Check sheet for the modelled part. Datum: model origin and axes. Units: mm. A direction names the side the tool comes from. Give positions to 0.01 mm unless a question says otherwise; leave off trailing zeros. Order: outer loops, then holes, each group sorted by start corner. A loop starts at its lowest first (then second) coordinate and runs counter-clockwise, first axis right, second up. Notation, with made-up numbers: (33.5, -31) -> (37.5, -31) arc R23 cw to (37.5, -19) -> close; hole circle Ø2 at (19, 12.5). An arc over 180 degrees is marked (long way). Answer in a Markdown table with one row per item. Add a question column.
(1) Cross-section at B-B (y = 0). Record the cut outline in (x, z).
(2) Release check for a two-part mould opening along Z. For faces 6 (the face through (-4.3, 4.5, 4.5)), 7 (the face through (0, 8, 3)), 8 (the face through (0.56, 6.14, 7)) record: released by +Z, released by -Z, zero draft, split by the parting line, or undercut.
(3) Cross-section at A-A (z = 3.5). Record the cut outline in (x, y).
(4) Set-up check for faces 1 (the face through (0, 4.5, -7)), 2 (the face through (-1.25, 7, 3)), 3 (the face through (7, 1.25, 3)), 4 (the face through (0, -1.25, 2)), 5 (the face through (-4.9, 5, 5.8)): record each of +Z, -Z, +X, -X, +Y, -Y from which the full face is reachable in a straight line by a thin tool's end or side.
(5) Cross-section at D-D (x = 0). Record the cut outline in (y, z), then the cut area to 3 significant figures.
(6) Cross-section at C-C (x = -6.5). Record the cut outline in (y, z), then the cut area to 3 significant figures.
(7) Go/stop test with flat-tipped pins: pin 1 (3 mm diameter, centred on x = -5.5, y = 5, fed in from -Z); pin 2 (2.5 mm diameter, centred on x = -0.5, y = 7.5, fed in from -Z); pin 3 (1.8 mm diameter, centred on x = 0.5, z = -8.5, fed in from +Y). Record where each tip stops, or that it passes through.
(8) Thickness scan on L1, parallel to Z at x = 4, y = 3.75; L2, parallel to Z at x = 3, y = 5.75; L3, parallel to Z at x = 2.5, y = 3.25. Record the ranges inside material, lowest first. Write a range as [from, to].
```python
from build123d import *
from build123d.topology import SkipClean

# Parameters (mm, degrees)
BOSS_EXTRUDE1_DEPTH = 7
BOSS_EXTRUDE2_DEPTH = 16
BOSS_EXTRUDE3_START = -16
BOSS_EXTRUDE3_DEPTH = 2.5
BOSS_EXTRUDE4_START = -5
BOSS_EXTRUDE4_DEPTH = 2.5
CUT_EXTRUDE1_START  = -7
SKETCH7_R           = 7.581765893
CUT_EXTRUDE1_DEPTH  = 7
BOSS_EXTRUDE5_START = 3
BOSS_EXTRUDE5_DEPTH = 3
BOSS_EXTRUDE6_DEPTH = 8
BOSS_EXTRUDE7_DEPTH = 8


with BuildPart() as part:
    # Sketch1 → Boss-Extrude1 (new body)
    with BuildSketch(Plane.XY):
        with BuildLine():
            Line((8, 1.25), (5.868347297, 1.25))
            ThreePointArc((5.868347297, 1.25), (4.242640687, 4.242640687), (1.25, 5.868347297))
            Line((1.25, 5.868347297), (1.25, 8))
            Line((1.25, 8), (-1.25, 8))
            Line((-1.25, 8), (-1.25, 5.868347297))
            ThreePointArc((-1.25, 5.868347297), (-4.242640687, 4.242640687), (-5.868347297, 1.25))
            Line((-5.868347297, 1.25), (-8, 1.25))
            Line((-8, 1.25), (-8, -1.25))
            Line((-8, -1.25), (8, -1.25))
            Line((8, -1.25), (8, 1.25))
        make_face()
    extrude(amount=BOSS_EXTRUDE1_DEPTH)

    # Sketch3 → Boss-Extrude2 (add)
    with BuildSketch(Plane.XY.offset(7)):
        with BuildLine():
            Line((-5.868347297, -1.25), (5.868347297, -1.25))
            ThreePointArc((5.868347297, -1.25), (0, 6), (-5.868347297, -1.25))
        make_face()
    extrude(amount=BOSS_EXTRUDE2_DEPTH)

    # Sketch5 → Boss-Extrude3 (add)
    with BuildSketch(Plane.XY.offset(23).offset(BOSS_EXTRUDE3_START)):
        with BuildLine():
            Line((-6.887488657, -1.25), (6.887488657, -1.25))
            ThreePointArc((6.887488657, -1.25), (0, 7), (-6.887488657, -1.25))
        make_face()
    extrude(amount=-BOSS_EXTRUDE3_DEPTH)

    # Sketch6 → Boss-Extrude4 (add)
    with BuildSketch(Plane.XY.offset(23).offset(BOSS_EXTRUDE4_START)):
        with BuildLine():
            Line((-6.887488657, -1.25), (6.887488657, -1.25))
            ThreePointArc((6.887488657, -1.25), (0, 7), (-6.887488657, -1.25))
        make_face()
    extrude(amount=-BOSS_EXTRUDE4_DEPTH)

    # Sketch7 → Cut-Extrude1 (cut)
    with BuildSketch(Plane.XY.offset(23).offset(CUT_EXTRUDE1_START)):
        Circle(SKETCH7_R)
        with BuildLine():
            Line((-4.841229183, -1.25), (4.841229183, -1.25))
            ThreePointArc((4.841229183, -1.25), (0, 5), (-4.841229183, -1.25))
        make_face(mode=Mode.SUBTRACT)
    extrude(amount=-CUT_EXTRUDE1_DEPTH, mode=Mode.SUBTRACT)

    # Sketch8 → Boss-Extrude5 (add)
    with SkipClean():  # the faces are left unmerged after this step: merging them gives an invalid solid
        with BuildSketch(Plane(origin=(0, 0, 0), x_dir=(-1, 0, 0), z_dir=(0, 0, -1)).offset(BOSS_EXTRUDE5_START)):
            with BuildLine():
                Line((-5.868347297, -1.25), (5.868347297, -1.25))
                ThreePointArc((5.868347297, -1.25), (0, 6), (-5.868347297, -1.25))
            make_face()
        extrude(amount=-BOSS_EXTRUDE5_DEPTH)

    # Sketch9 → Boss-Extrude6 (add)
    with SkipClean():  # the faces are left unmerged after this step: merging them gives an invalid solid
        with BuildSketch(Plane(origin=(0, 0, -3), x_dir=(-1, 0, 0), z_dir=(0, 0, -1))):
            with BuildLine():
                Line((-3.588523373, -1.25), (3.588523373, -1.25))
                ThreePointArc((3.588523373, -1.25), (3.321506513, 1.845967087), (0.833333333, 3.707499906))
                Line((0.833333333, 3.707499906), (0.833333333, 4.5))
                Line((0.833333333, 4.5), (-0.833333333, 4.5))
                Line((-0.833333333, 4.5), (-0.833333333, 3.707499906))
                ThreePointArc((-0.833333333, 3.707499906), (-3.321506513, 1.845967087), (-3.588523373, -1.25))
            make_face()
        extrude(amount=BOSS_EXTRUDE6_DEPTH)

    # Sketch10 → Boss-Extrude7 (add)
    with SkipClean():  # the faces are left unmerged after this step: merging them gives an invalid solid
        with BuildSketch(Plane(origin=(0, 0, -11), x_dir=(-1, 0, 0), z_dir=(0, 0, -1))):
            with BuildLine():
                Line((-3.588523373, -1.25), (3.588523373, -1.25))
                ThreePointArc((3.588523373, -1.25), (0, 3.8), (-3.588523373, -1.25))
            make_face()
        extrude(amount=BOSS_EXTRUDE7_DEPTH)


solid = part.part
```
Answer below:
| question | item | result |
|---|---|---|
| 1 | outline | (-8, 0) -> (-6, 0) -> (-6, -3) -> (-3.8, -3) -> (-3.8, -19) -> (3.8, -19) -> (3.8, -3) -> (6, -3) -> (6, 0) -> (8, 0) -> (8, 7) -> (6, 7) -> (6, 9) -> (5, 9) -> (5, 16) -> (7, 16) -> (7, 18) -> (6, 18) -> (6, 23) -> (-6, 23) -> (-6, 18) -> (-7, 18) -> (-7, 16) -> (-5, 16) -> (-5, 9) -> (-6, 9) -> (-6, 7) -> (-8, 7) -> close |
| 2 | face 6 | released by -Z |
| 2 | face 7 | zero draft |
| 2 | face 8 | undercut |
| 3 | outline | (-8, -1.25) -> (8, -1.25) -> (8, 1.25) -> (5.87, 1.25) arc R6 ccw to (1.25, 5.87) -> (1.25, 8) -> (-1.25, 8) -> (-1.25, 5.87) arc R6 ccw to (-5.87, 1.25) -> (-8, 1.25) -> close |
| 4 | face 1 | -Z, +X, -X, +Y |
| 4 | face 2 | -Z, -X, +Y |
| 4 | face 3 | -Z, +X, +Y |
| 4 | face 4 | +Z, -Z, +X, -X, -Y |
| 4 | face 5 | +Z, -Z, -X, +Y |
| 5 | outline | (-1.25, -19) -> (3.8, -19) -> (3.8, -11) -> (4.5, -11) -> (4.5, -3) -> (6, -3) -> (6, 0) -> (8, 0) -> (8, 7) -> (6, 7) -> (6, 9) -> (5, 9) -> (5, 16) -> (7, 16) -> (7, 18) -> (6, 18) -> (6, 23) -> (-1.25, 23) -> close |
| 5 | area | 284 mm² |
| 6 | outline | (-1.25, 0) -> (1.25, 0) -> (1.25, 4.5) -> (2.6, 4.5) -> (2.6, 7) -> (-1.25, 7) -> close; (-1.25, 16) -> (2.6, 16) -> (2.6, 18) -> (-1.25, 18) -> close |
| 6 | area | 28.6 mm² |
| 7 | pin 1 | stops at z = -3 |
| 7 | pin 2 | stops at z = 0 |
| 7 | pin 3 | stops at y = 4.5 |
| 8 | L1 | z = [-3, 9], [16, 23] |
| 8 | L2 | z = [4.5, 7], [16, 18] |
| 8 | L3 | z = [-3, 23] |
